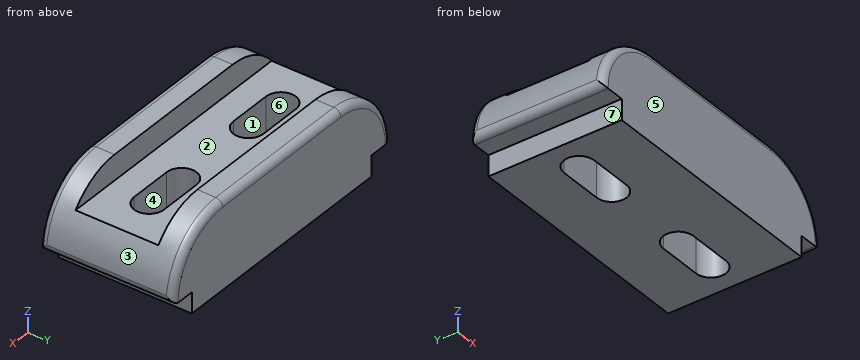
from build123d import *

# Parameters (mm, degrees)
F1_DEPTH = 58
F3_W     = 36
F3_H     = 11
F4_DEPTH = 127
F6_DEPTH = 38
F7_R     = 3


with BuildPart() as f1:
    # F0 (on Front) → F1 (new body)
    with BuildSketch(Plane.XZ):
        with BuildLine():
            Line((0, 9), (0, 0))
            Line((0, 0), (105, 0))
            Line((105, 0), (105, 9))
            Line((105, 9), (116, 9))
            ThreePointArc((116, 9), (107.506097, 29.506097), (87, 38))
            Line((87, 38), (18, 38))
            ThreePointArc((18, 38), (-2.506097, 29.506097), (-11, 9))
            Line((-11, 9), (0, 9))
        make_face()
    extrude(amount=-F1_DEPTH)

    # F3 (on offset) → F4 (cut)
    with BuildSketch(Plane.YZ.offset(-11)):
        with Locations((29, 32.5)):
            Rectangle(F3_W, F3_H)
    extrude(amount=F4_DEPTH, mode=Mode.SUBTRACT)

    # F5 (on face) → F6 (cut)
    with BuildSketch(Plane.XY.offset(27)):
        with BuildLine():
            Line((33, 35.5), (14, 35.5))
            ThreePointArc((14, 35.5), (7.5, 29), (14, 22.5))
            Line((14, 22.5), (33, 22.5))
            ThreePointArc((33, 22.5), (39.5, 29), (33, 35.5))
        make_face()
        with BuildLine():
            Line((72, 22.5), (91, 22.5))
            ThreePointArc((91, 22.5), (97.5, 29), (91, 35.5))
            Line((91, 35.5), (72, 35.5))
            ThreePointArc((72, 35.5), (65.5, 29), (72, 22.5))
        make_face()
    extrude(amount=-F6_DEPTH, mode=Mode.SUBTRACT)

    # F7
    f7_edges = [f1.edges().sort_by_distance(p)[0] for p in [
        (107.506097, 0, 29.506097),
        (116, 29, 9),
        (107.506097, 58, 29.506097),
        (-11, 29, 9),
    ]]
    fillet(f7_edges, radius=F7_R)


solid = f1.part
Build history of the part. All positions in model axes, mm. Face numbers are marked on the shaded views. A direction names the side the tool comes from. Give positions to 0.01 mm unless a question says otherwise; leave off trailing zeros. Order: outer loops, then holes, each group sorted by start corner. A loop starts at its lowest first (then second) coordinate and runs counter-clockwise, first axis right, second up. Notation, with made-up numbers: M 87,12 L 117,12 A15 ccw 117,23 Z; hole C 19,68 d5. An arc over 180 degrees is marked long. Put each result on its own line as item: value.
Item 1: Drop flat-ended pins along their axis: pin 1 Ø10 at (y, z) = (6.5, 18.5) entering from -X; pin 2 Ø10 at (y, z) = (26.5, 6.5) entering from -X; pin 3 Ø6.5 at (x, y) = (108.5, 16) entering from -Z. Give the stop position or say it passes through.
Results are:
pin 1: x = -10.65
pin 2: x = -10.78
pin 3: z = 9
Item 2: Which spindle directions (+Z, -Z, +X, -X, +Y, -Y) get a long thin tool onto all of the face, cutting with end or side? Do the marked faces 1, 2 and 3. Say none if no direction does.
Results are:
face 1: +Z, -Z
face 2: +Z, +X, -X
face 3: +Z, +X, +Y, -Y
Item 3: Cut at B-B on y = 29. Write the cut outline in (x, z).
Results are:
outline: M -10.81,12.35 A3 ccw -7.83,9 L 0,9 L 0,0 L 7.5,0 L 7.5,27 L -4.74,27 A29 ccw Z; M 39.5,0 L 65.5,0 L 65.5,27 L 39.5,27 Z; M 97.5,0 L 105,0 L 105,9 L 112.83,9 A3 ccw 115.81,12.35 A29 ccw 109.74,27 L 97.5,27 Z
Item 4: Cut at A-A on x = 22. Write the cut outline in (y, z), then the cut area to 3 significant figures.
Results are:
outline: M 0,0 L 22.5,0 L 22.5,27 L 11,27 L 11,38 L 3,38 A3 ccw 0,35 Z; M 35.5,0 L 58,0 L 58,35 A3 ccw 55,38 L 47,38 L 47,27 L 35.5,27 Z
area: 1,450 mm2
Item 5: Cut at C-C on y = 49. Write the cut outline in (x, z), then the cut area to 3 significant figures.
Results are:
outline: M -10.81,12.35 A3 ccw -7.83,9 L 0,9 L 0,0 L 105,0 L 105,9 L 112.83,9 A3 ccw 115.81,12.35 A29 ccw 87,38 L 18,38 A29 ccw Z
area: 4,260 mm2
Item 6: Pull direction Y, two halves, no side cores. Call the marked faces 4, 5, 6 and 7: +Y half, -Y half, draft (parallel to the pull), parting line (faces both ways), or undercut.
Results are:
face 4: undercut
face 5: -Y half
face 6: undercut
face 7: draft
Item 7: Cut at D-D on x = 45.5. Write the cut outline in (y, z), then the cut area to 3 significant figures.
Results are:
outline: M 0,0 L 58,0 L 58,35 A3 ccw 55,38 L 47,38 L 47,27 L 11,27 L 11,38 L 3,38 A3 ccw 0,35 Z
area: 1,800 mm2
Item 8: Wall check: probe 1 along Y at (x, z) = (29, 5); probe 2 along X at (y, z) = (35, 13); probe 3 along Y at (x, z) = (96, 32). Give the ranges that are in metal, low to high.
Results are:
probe 1: 0 to 22.5, 35.5 to 58
probe 2: -10.72 to 11.5, 35.5 to 69.5, 93.5 to 115.72
probe 3: 0 to 11, 47 to 58
